```python
from build123d import *

# Parameters (mm, degrees)
SKETCH1_W           = 30
SKETCH1_H           = 9
BOSS_EXTRUDE1_DEPTH = 22.7
SKETCH3_R           = 9
BOSS_EXTRUDE2_DEPTH = 28.5
SKETCH4_R           = 8.25
BOSS_EXTRUDE3_DEPTH = 40
SKETCH5_W           = 3.25
SKETCH5_H           = 1.5
CUT_EXTRUDE1_DEPTH  = 20
CHAMFER1_SIZE       = 0.5


with BuildPart() as part:
    # Sketch1 → Revolve1 (revolve)
    with BuildSketch(Plane.XY, mode=Mode.PRIVATE) as revolve1_sk:
        with Locations((15, 4.5)):
            Rectangle(SKETCH1_W, SKETCH1_H)
    revolve(revolve1_sk.sketch.rotate(Axis((0, 0, 0), (1, 0, 0)), 90), axis=Axis((0, 0, 0), (1, 0, 0)))

    # Sketch2 → Boss-Extrude1 (add)
    with BuildSketch(Plane(origin=(30, 0, 0), x_dir=(0, 0, -1), z_dir=(1, 0, 0))):
        with BuildLine():
            Line((-5, 18.142135624), (5, 18.142135624))
            Line((5, 18.142135624), (5, 14.142135624))
            ThreePointArc((5, 14.142135624), (0, -15), (-5, 14.142135624))
            Line((-5, 14.142135624), (-5, 18.142135624))
        make_face()
    extrude(amount=BOSS_EXTRUDE1_DEPTH)

    # Sketch3 → Boss-Extrude2 (add)
    with BuildSketch(Plane(origin=(52.7, 0, 0), x_dir=(0, 0, -1), z_dir=(1, 0, 0))):
        with Locations(Location((0, 0, 0), (0, 0, 180))):
            Circle(SKETCH3_R)
    extrude(amount=BOSS_EXTRUDE2_DEPTH)

    # Sketch4 → Boss-Extrude3 (add)
    with BuildSketch(Plane(origin=(81.2, 0, 0), x_dir=(0, 0, -1), z_dir=(1, 0, 0))):
        Circle(SKETCH4_R)
    extrude(amount=BOSS_EXTRUDE3_DEPTH)

    # Sketch5 → Cut-Extrude1 (cut)
    with BuildSketch(Plane(origin=(121.2, 0, 0), x_dir=(0, 0, -1), z_dir=(1, 0, 0))):
        with Locations((0, 7.79)):
            Rectangle(SKETCH5_W, SKETCH5_H)
    extrude(amount=-CUT_EXTRUDE1_DEPTH, mode=Mode.SUBTRACT)

    # Chamfer1
    chamfer1_edges = [part.edges().sort_by_distance(p)[0] for p in [
        (0, 0, -9),
    ]]
    chamfer(chamfer1_edges, length=CHAMFER1_SIZE)


solid = part.part
```
Could you check a few things on this model? Use its own coordinates, in mm. A direction names the side the tool comes from. Give positions to 0.01 mm unless a question says otherwise; leave off trailing zeros. Order: outer loops, then holes, each group sorted by start corner. A loop starts at its lowest first (then second) coordinate and runs counter-clockwise, first axis right, second up.
Q1. Suppose I cut it at A-A, the plane y = 0. Write out the boundary of the cut face in (x, z).
Q2. If I drill on line 1 along X through (y, z) = (11.5, -2); line 2 along Y through (x, z) = (27, 3); line 3 along Y through (x, z) = (38.5, -0.5), over which ranges is the centre line in solid material (lowest first)?
Q3. Suppose I cut it at C-C, the plane x = 38. Write out the boundary of the cut face in (y, z).
Q4. For faces 1 (the cylindrical face through (15.456, -6.083, -6.633)), 2 (the flat face through (52.7, 9.2, -0.2)), 3 (the flat face through (41, 16, -5)), 4 (the flat face through (111, 7.04, 0)), 5 (the flat face through (41, 16, 5)), which set-ups out of +Z, -Z, +X, -X, +Y, -Y let a thin tool reach every point of the face, with its end or its side?
Q5. Suppose I cut it at B-B, the plane z = 0. Write out the boundary of the cut face in (x, y).
Q6. Suppose I cut it at D-D, the plane y = 15.5. Write out the boundary of the cut face in (x, z).
Q7. I'm going to push flat-ended pins straight in: P1, Ø10, axis at x = 96, z = 3.5, coming from the -Y side; P2, Ø8, axis at x = 81.5, z = -4.5, coming from the +Y side; P3, Ø0.5, axis at x = 114, y = 7.5, coming from the -Z side. Where does each tip first touch, or does it pass through?
Solution:
1. outline: (0, -8.5) - (0.5, -9) - (30, -9) - (30, -15) - (52.7, -15) - (52.7, -9) - (81.2, -9) - (81.2, -8.25) - (121.2, -8.25) - (121.2, 8.25) - (81.2, 8.25) - (81.2, 9) - (52.7, 9) - (52.7, 15) - (30, 15) - (30, 9) - (0.5, 9) - (0, 8.5) - close
2. line 1: x = 30 to 52.7
2. line 2: y = -8.49 to 8.49
2. line 3: y = -14.99 to 18.14
3. outline: (14.14, -5) - (18.14, -5) - (18.14, 5) - (14.14, 5) arc R15 ccw (long way) to start
4. face 1: -X
4. face 2: +X
4. face 3: -Z, +X, -X, +Y
4. face 4: +X, +Y
4. face 5: +Z, +X, -X, +Y
5. outline: (0, -8.5) - (0.5, -9) - (30, -9) - (30, -15) - (52.7, -15) - (52.7, -9) - (81.2, -9) - (81.2, -8.25) - (121.2, -8.25) - (121.2, 7.04) - (101.2, 7.04) - (101.2, 8.25) - (81.2, 8.25) - (81.2, 9) - (52.7, 9) - (52.7, 18.14) - (30, 18.14) - (30, 9) - (0.5, 9) - (0, 8.5) - close
6. outline: (30, -5) - (52.7, -5) - (52.7, 5) - (30, 5) - close
7. P1: stops at y = -8.25
7. P2: stops at y = 8.99
7. P3: stops at z = -3.94
